Source: CAD feature listing. Evaluate the final solid. Frame: model axes, mm. Give positions to 0.01 mm unless a question says otherwise; leave off trailing zeros.
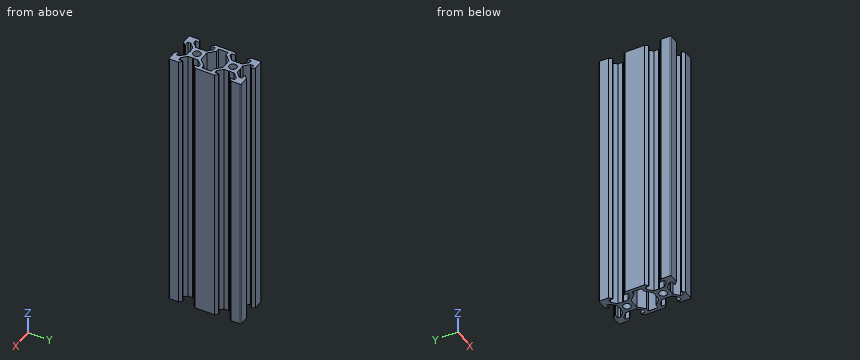
```python
from build123d import *

# Parameters (mm, degrees)
SKETCH1_R           = 2.1
BOSS_EXTRUDE1_DEPTH = 150


with BuildPart() as part:
    # Sketch1 → Boss-Extrude1 (new body)
    with BuildSketch(Plane.XY):
        with BuildLine():
            Line((4.58, -20), (9.5, -20))
            ThreePointArc((9.5, -20), (9.853553391, -19.853553391), (10, -19.5))
            Line((10, -19.5), (10, -14.58))
            Line((10, -14.58), (8.545, -13.125))
            Line((8.545, -13.125), (8.2, -13.125))
            Line((8.2, -13.125), (8.2, -15.5))
            Line((8.2, -15.5), (6.560660172, -15.5))
            Line((6.560660172, -15.5), (3.9, -12.839339828))
            Line((3.9, -12.839339828), (3.9, -10.21))
            Line((3.9, -10.21), (3.69, -10))
            Line((3.69, -10), (3.9, -9.79))
            Line((3.9, -9.79), (3.9, -7.160660172))
            Line((3.9, -7.160660172), (6.560660172, -4.5))
            Line((6.560660172, -4.5), (8.2, -4.5))
            Line((8.2, -4.5), (8.2, -6.875))
            Line((8.2, -6.875), (8.545, -6.875))
            Line((8.545, -6.875), (10, -5.42))
            Line((10, -5.42), (10, 5.42))
            Line((10, 5.42), (8.545, 6.875))
            Line((8.545, 6.875), (8.2, 6.875))
            Line((8.2, 6.875), (8.2, 4.5))
            Line((8.2, 4.5), (6.560660172, 4.5))
            Line((6.560660172, 4.5), (3.9, 7.160660172))
            Line((3.9, 7.160660172), (3.9, 9.79))
            Line((3.9, 9.79), (3.69, 10))
            Line((3.69, 10), (3.9, 10.21))
            Line((3.9, 10.21), (3.9, 12.839339828))
            Line((3.9, 12.839339828), (6.560660172, 15.5))
            Line((6.560660172, 15.5), (8.2, 15.5))
            Line((8.2, 15.5), (8.2, 13.125))
            Line((8.2, 13.125), (8.545, 13.125))
            Line((8.545, 13.125), (10, 14.58))
            Line((10, 14.58), (10, 19.5))
            ThreePointArc((10, 19.5), (9.853553391, 19.853553391), (9.5, 20))
            Line((9.5, 20), (4.58, 20))
            Line((4.58, 20), (3.125, 18.545))
            Line((3.125, 18.545), (3.125, 18.2))
            Line((3.125, 18.2), (5.5, 18.2))
            Line((5.5, 18.2), (5.5, 16.560660172))
            Line((5.5, 16.560660172), (2.839339828, 13.9))
            Line((2.839339828, 13.9), (0.21, 13.9))
            Line((0.21, 13.9), (0, 13.69))
            Line((0, 13.69), (-0.21, 13.9))
            Line((-0.21, 13.9), (-2.839339828, 13.9))
            Line((-2.839339828, 13.9), (-5.5, 16.560660172))
            Line((-5.5, 16.560660172), (-5.5, 18.2))
            Line((-5.5, 18.2), (-3.125, 18.2))
            Line((-3.125, 18.2), (-3.125, 18.545))
            Line((-3.125, 18.545), (-4.58, 20))
            Line((-4.58, 20), (-9.5, 20))
            ThreePointArc((-9.5, 20), (-9.853553391, 19.853553391), (-10, 19.5))
            Line((-10, 19.5), (-10, 14.58))
            Line((-10, 14.58), (-8.545, 13.125))
            Line((-8.545, 13.125), (-8.2, 13.125))
            Line((-8.2, 13.125), (-8.2, 15.5))
            Line((-8.2, 15.5), (-6.560660172, 15.5))
            Line((-6.560660172, 15.5), (-3.9, 12.839339828))
            Line((-3.9, 12.839339828), (-3.9, 10.21))
            Line((-3.9, 10.21), (-3.69, 10))
            Line((-3.69, 10), (-3.9, 9.79))
            Line((-3.9, 9.79), (-3.9, 7.160660172))
            Line((-3.9, 7.160660172), (-6.560660172, 4.5))
            Line((-6.560660172, 4.5), (-8.2, 4.5))
            Line((-8.2, 4.5), (-8.2, 6.875))
            Line((-8.2, 6.875), (-8.545, 6.875))
            Line((-8.545, 6.875), (-10, 5.42))
            Line((-10, 5.42), (-10, -5.42))
            Line((-10, -5.42), (-8.545, -6.875))
            Line((-8.545, -6.875), (-8.2, -6.875))
            Line((-8.2, -6.875), (-8.2, -4.5))
            Line((-8.2, -4.5), (-6.560660172, -4.5))
            Line((-6.560660172, -4.5), (-3.9, -7.160660172))
            Line((-3.9, -7.160660172), (-3.9, -9.79))
            Line((-3.9, -9.79), (-3.69, -10))
            Line((-3.69, -10), (-3.9, -10.21))
            Line((-3.9, -10.21), (-3.9, -12.839339828))
            Line((-3.9, -12.839339828), (-6.560660172, -15.5))
            Line((-6.560660172, -15.5), (-8.2, -15.5))
            Line((-8.2, -15.5), (-8.2, -13.125))
            Line((-8.2, -13.125), (-8.545, -13.125))
            Line((-8.545, -13.125), (-10, -14.58))
            Line((-10, -14.58), (-10, -19.5))
            ThreePointArc((-10, -19.5), (-9.853553391, -19.853553391), (-9.5, -20))
            Line((-9.5, -20), (-4.58, -20))
            Line((-4.58, -20), (-3.125, -18.545))
            Line((-3.125, -18.545), (-3.125, -18.2))
            Line((-3.125, -18.2), (-5.5, -18.2))
            Line((-5.5, -18.2), (-5.5, -16.560660172))
            Line((-5.5, -16.560660172), (-2.839339828, -13.9))
            Line((-2.839339828, -13.9), (-0.21, -13.9))
            Line((-0.21, -13.9), (0, -13.69))
            Line((0, -13.69), (0.21, -13.9))
            Line((0.21, -13.9), (2.839339828, -13.9))
            Line((2.839339828, -13.9), (5.5, -16.560660172))
            Line((5.5, -16.560660172), (5.5, -18.2))
            Line((5.5, -18.2), (3.125, -18.2))
            Line((3.125, -18.2), (3.125, -18.545))
            Line((3.125, -18.545), (4.58, -20))
        make_face()
        with Locations((0, -10)):
            Circle(SKETCH1_R, mode=Mode.SUBTRACT)
        Polygon((-6.239339828, -2.7), (-8.2, -2.7), (-8.2, 2.7), (-6.239339828, 2.7), (-2.839339828, 6.1), (2.839339828, 6.1), (6.239339828, 2.7), (8.2, 2.7), (8.2, -2.7), (6.239339828, -2.7), (2.839339828, -6.1), (-2.839339828, -6.1), align=None, mode=Mode.SUBTRACT)
        with Locations((0, 10)):
            Circle(SKETCH1_R, mode=Mode.SUBTRACT)
    extrude(amount=BOSS_EXTRUDE1_DEPTH)


solid = part.part
```
1) Material intervals for L1, parallel to Y at x = 0, z = 91; L2, parallel to Y at x = -0.25, z = 9; L3, parallel to Y at x = -2.25, z = 55, sorted ascending.
Report:
L1: y = -13.69 to -12.1, -7.9 to -6.1, 6.1 to 7.9, 12.1 to 13.69
L2: y = -13.9 to -12.09, -7.91 to -6.1, 6.1 to 7.91, 12.09 to 13.9
L3: y = -13.9 to -6.1, 6.1 to 13.9
2) Pin query (flat end, axial travel): pin 1 (3 mm diameter, centred on y = 8, z = 62.5, fed in from -X); pin 2 (1 mm diameter, centred on x = -3.5, y = -4, fed in from -Z); pin 3 (2 mm diameter, centred on x = 2, z = 89.5, fed in from +Y). Return the tip coordinate at first contact, or that it passes through.
Report:
pin 1: stops at x = -8.92
pin 2: passes through
pin 3: stops at y = 14.06
3) Section query A-A, the plane z = 126. Count the separate pieces of the cut face and the enclosed holes in it, and give its area (3 significant figures).
Report:
separate pieces: 1
enclosed holes: 3
area: 300 mm2
